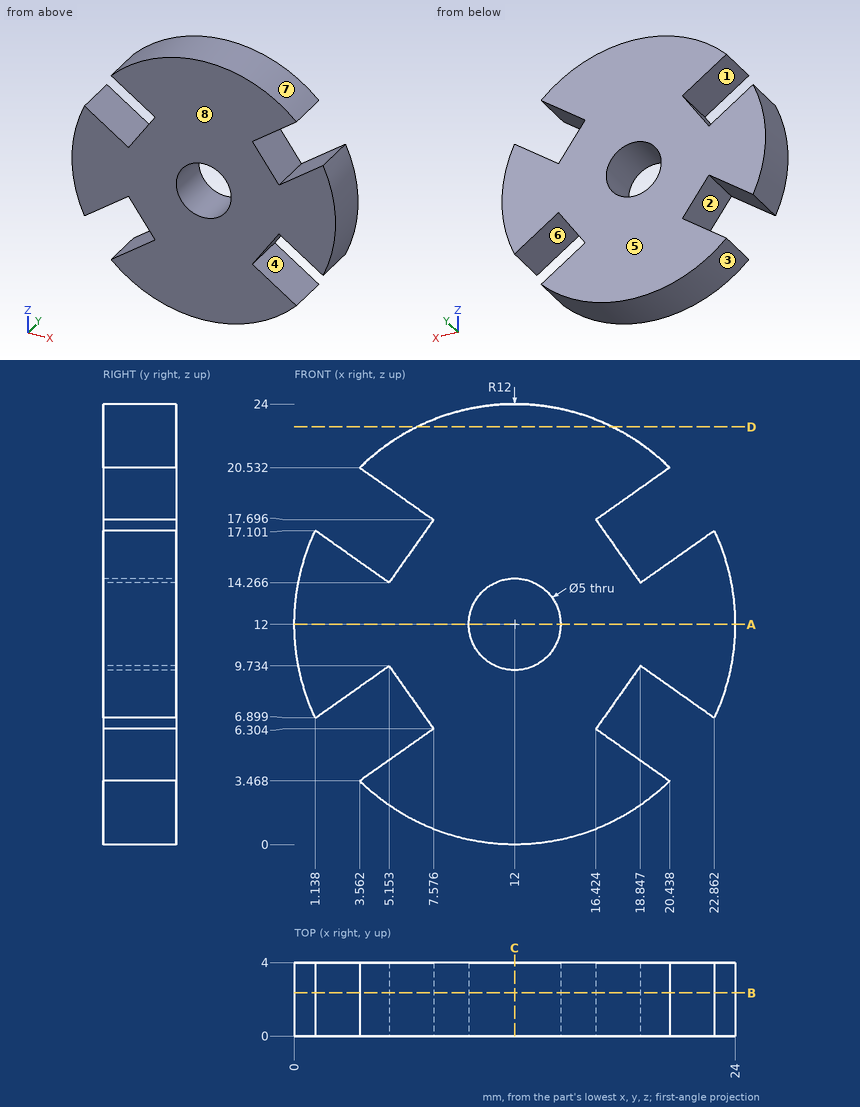
For this review, use the dimensioned drawing (mm, ordinates from the lowest corner) and the shaded views. A direction names the side the tool comes from. Give positions to 0.01 mm unless a question says otherwise; leave off trailing zeros. Write each loop counter-clockwise with the first axis right and the second up, starting at its lowest first coordinate (ties: lowest second). Pieces come first, ordered by that corner, then holes.
(1) The part is to be moulded in two halves that separate along Z. For the marked faces 6, 7 and 8, say which applies: released by +Z, released by -Z, zero draft, split by the parting line, or undercut.
(2) Consider section D-D, the plane z = 22.75. Give the boundary of the cut face in (x, y).
(3) Tool access review of the marked faces 1, 2, 3, 4 and 5: name each direction out of +Z, -Z, +X, -X, +Y, -Y from which nothing blocks a thin tool from reaching the whole face with its end or side.
(4) Consider section A-A, the plane z = 12. Give the boundary of the cut face in (x, y), and give its area (3 significant figures).
(5) To check wall thickness, follow L1, parallel to Z at x = 19, y = 1.85 (1 decimal); L2, parallel to Z at x = 7, y = 3.6 (1 decimal); L3, parallel to X at y = 1.55, z = 16.5 (1 decimal). State the ranges of each line that lie inside material, in increasing order.
(6) Consider section B-B, the plane y = 2.35. Give the boundary of the cut face in (x, z) (1 decimal), and give its area (3 significant figures).
(7) For P1, Ø4, axis at x = 12, z = 12, coming from the +Y side, flat-tipped, find the tip position at first contact; note if it passes through.
(8) Consider section C-C, the plane x = 12. Give the boundary of the cut face in (y, z).
Returned:
1. face 6: undercut
1. face 7: released by +Z
1. face 8: zero draft
2. outline: (6.67, 0) - (17.33, 0) - (17.33, 4) - (6.67, 4) - close
3. face 1: -X, +Y, -Y
3. face 2: +Y, -Y
3. face 3: -Z, +Y, -Y
3. face 4: +X, +Y, -Y
3. face 5: +Z, -Z, +X, -X, +Y
4. outline: (0, 0) - (9.5, 0) - (9.5, 4) - (0, 4) - close; (14.5, 0) - (24, 0) - (24, 4) - (14.5, 4) - close
4. area: 76.0 mm2
5. L1: z = 2.3 to 4.5, 9.6 to 14.4, 19.5 to 21.7
5. L2: z = 1.1 to 5.9, 7.1 to 16.9, 18.1 to 22.9
5. L3: x = 0.9 to 2, 6.7 to 17.3, 22 to 23.1
6. outline: (1.1, 6.9) - (5.2, 9.7) - (7.6, 6.3) - (3.6, 3.5) arc R12 ccw to (20.4, 3.5) - (16.4, 6.3) - (18.8, 9.7) - (22.9, 6.9) arc R12 ccw to (22.9, 17.1) - (18.8, 14.3) - (16.4, 17.7) - (20.4, 20.5) arc R12 ccw to (3.6, 20.5) - (7.6, 17.7) - (5.2, 14.3) - (1.1, 17.1) arc R12 ccw to start; hole circle Ø5 at (12, 12)
6. area: 348 mm2
7. P1: passes through
8. outline: (0, 0) - (4, 0) - (4, 9.5) - (0, 9.5) - close; (0, 14.5) - (4, 14.5) - (4, 24) - (0, 24) - close
